```python
from build123d import *

# Parameters (mm, degrees)
F1_DEPTH = 30.48
F3_DEPTH = 0.762


with BuildPart() as f1:
    # F0 (on Front) → F1 (new body)
    with BuildSketch(Plane.XZ):
        with BuildLine():
            Line((-8.5725, 0), (8.5725, 0))
            ThreePointArc((8.5725, 0), (8.082949, 2.855468), (6.670209, 5.3848))
            Line((6.670209, 5.3848), (-6.670209, 5.3848))
            ThreePointArc((-6.670209, 5.3848), (-8.082949, 2.855468), (-8.5725, 0))
        make_face()
        with BuildLine():
            ThreePointArc((-7.684708, 1.396131), (-7.173881, 3.088582), (-6.295525, 4.6228))
            Line((-6.295525, 4.6228), (6.295525, 4.6228))
            ThreePointArc((6.295525, 4.6228), (7.177049, 3.081214), (7.687559, 1.380345))
            Line((7.687559, 1.380345), (7.874, 1.380345))
            Line((7.874, 1.380345), (7.874, 0.762))
            Line((7.874, 0.762), (7.77324, 0.762))
            Line((7.77324, 0.762), (-7.77324, 0.762))
            Line((-7.77324, 0.762), (-7.874, 0.762))
            Line((-7.874, 0.762), (-7.874, 1.396131))
            Line((-7.874, 1.396131), (-7.684708, 1.396131))
        make_face(mode=Mode.SUBTRACT)
    extrude(amount=-F1_DEPTH)

    # F2 (on face) → F3 (join)
    with BuildSketch(Plane.XZ):
        with BuildLine():
            ThreePointArc((-6.295525, 4.6228), (-7.173881, 3.088582), (-7.684708, 1.396131))
            Line((-7.684708, 1.396131), (-7.874, 1.396131))
            Line((-7.874, 1.396131), (-7.874, 0.762))
            Line((-7.874, 0.762), (7.874, 0.762))
            Line((7.874, 0.762), (7.874, 1.380345))
            Line((7.874, 1.380345), (7.687559, 1.380345))
            ThreePointArc((7.687559, 1.380345), (7.177049, 3.081214), (6.295525, 4.6228))
            Line((6.295525, 4.6228), (-6.295525, 4.6228))
        make_face()
    extrude(amount=-F3_DEPTH)


solid = f1.part
```
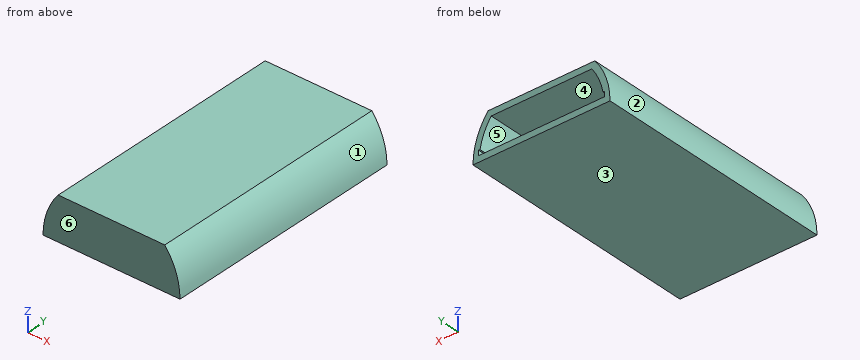
Source: CAD feature listing. Evaluate the final solid. Frame: model axes, mm. Face numbers are marked on the shaded views. A direction names the side the tool comes from. Round coordinates to 2 decimals unless told otherwise and drop trailing zeros. Loops run counter-clockwise (first coordinate to the right, second up) from the corner with the lowest first, then second, coordinate; pieces in that order, holes last.
1. Mould query, pull axis X, two halves, no side actions, for the marked faces 1, 2, 3 and 4. Classes: released by +X, released by -X, zero draft, split by the parting line, or undercut.
2. Access query for the marked faces 5 and 6. Directions: +Z, -Z, +X, -X, +Y, -Y. A direction counts if a zero-diameter tool reaches every point of the face in a straight line with its end or side. Return the directions, or none.
3. Section query C-C on z = 2.35. Output: boundary loops of the cut face in (x, y).
4. Contact query for a flat-ended pin moving along its axis: pin 1 (1.5 mm diameter, centred on y = 14.5, z = 4.5, fed in from -X). Output: stop coordinate, or through.
5. Section query B-B on x = -2.5. Output: boundary loops of the cut face in (y, z), and give its area (3 significant figures).
6. Ray query, L1, parallel to Z at x = -2, y = 9; L2, parallel to Y at x = 5.75, z = 3.75; L3, parallel to X at y = 21.5, z = 3.8. Return the intervals inside material, ascending.
7. Section query D-D on z = 4.95. Output: boundary loops of the cut face in (x, y).
Answers below:
1. face 1: released by +X
1. face 2: released by -X
1. face 3: zero draft
1. face 4: undercut
2. face 5: +Y
2. face 6: +Z, -Z, +X, -X, -Y
3. outline: (-8.24, 0) - (8.24, 0) - (8.24, 30.48) - (7.45, 30.48) - (7.45, 0.76) - (-7.45, 0.76) - (-7.45, 30.48) - (-8.24, 30.48) - close
4. pin 1: stops at x = -7.71
5. outline: (0, 0) - (30.48, 0) - (30.48, 0.76) - (0.76, 0.76) - (0.76, 4.62) - (30.48, 4.62) - (30.48, 5.38) - (0, 5.38) - close
5. area: 49.4 mm2
6. L1: z = 0 to 0.76, 4.62 to 5.38
6. L2: y = 0 to 0.76
6. L3: x = -7.68 to -6.82, 6.82 to 7.68
7. outline: (-7, 0) - (7, 0) - (7, 30.48) - (-7, 30.48) - close
